from build123d import *

# Parameters (mm, degrees)
SKETCH1_W           = 9.849999945
SKETCH1_H           = 0.849999995
BOSS_EXTRUDE1_DEPTH = 10
BOSS_EXTRUDE2_DEPTH = 0.849999995
BOSS_EXTRUDE3_DEPTH = 0.150000005


with BuildPart() as part:
    # Sketch1 → Boss-Extrude1 (new body)
    with BuildSketch(Plane.XY):
        with Locations((2.94e-07, -2.739426966)):
            Rectangle(SKETCH1_W, SKETCH1_H)
    extrude(amount=BOSS_EXTRUDE1_DEPTH)

    # Sketch3 → Boss-Extrude2 (add)
    with BuildSketch(Plane.XZ.offset(3.164426964)):
        Polygon((-4.924999678, 0), (-4.924999678, 10), (-6.074999733, 10), (-6.074999733, 5.2), (-5.374999733, 4.6), (-5.374999733, 3.2), (-6.074999733, 3.2), (-6.074999733, 0), align=None)
    extrude(amount=-BOSS_EXTRUDE2_DEPTH)

    # Sketch4 → Boss-Extrude3 (add)
    with BuildSketch(Plane.XZ.offset(3.164426964)):
        with BuildLine():
            Line((-6.074999733, 10), (4.925000267, 10))
            Line((4.925000267, 10), (4.925000267, 8.5))
            ThreePointArc((4.925000267, 8.5), (-0.574999733, 8.25), (-6.074999733, 8.5))
            Line((-6.074999733, 8.5), (-6.074999733, 10))
        make_face()
    extrude(amount=BOSS_EXTRUDE3_DEPTH)


solid = part.part
Could you check a few things on this model? Use its own coordinates, in mm. Round coordinates to 2 decimals unless told otherwise and drop trailing zeros. Write each loop counter-clockwise with the first axis right and the second up, starting at its lowest first coordinate (ties: lowest second). Pieces come first, ordered by that corner, then holes. Notation, with made-up numbers: (24, 74) -> (71, 74) arc R23 ccw to (71, 103) -> close; hole circle Ø5 at (52, 11.25). An arc over 180 degrees is marked (long way). Use a Markdown table: item, result.
1. If we section it at D-D (x = -4.25): List the corners of the cut face in (y, z) for me, then the cut area to 3 significant figures.
Answer key:
| item | result |
|---|---|
| outline | (-3.31, 8.36) -> (-3.16, 8.36) -> (-3.16, 0) -> (-2.31, 0) -> (-2.31, 10) -> (-3.31, 10) -> close |
| area | 8.75 mm^2 |
2. If we section it at C-C (z = 6.5): List the corners of the cut face in (x, y) for me (3 decimals).
Answer key:
| item | result |
|---|---|
| outline | (-6.075, -3.164) -> (4.925, -3.164) -> (4.925, -2.314) -> (-6.075, -2.314) -> close |
3. If we section it at A-A (x = 1): List the corners of the cut face in (y, z) for me, then the cut area to 3 significant figures.
Answer key:
| item | result |
|---|---|
| outline | (-3.31, 8.27) -> (-3.16, 8.27) -> (-3.16, 0) -> (-2.31, 0) -> (-2.31, 10) -> (-3.31, 10) -> close |
| area | 8.76 mm^2 |
4. Please list where these lines run through material, in increasing order: probe 1 along Y at (x, z) = (-2.5, 4); probe 2 along Z at (x, y) = (-5.5, -2.7); probe 3 along X at (y, z) = (-3.1, 3.5) (3 decimals).
Answer key:
| item | result |
|---|---|
| probe 1 | y = -3.16 to -2.31 |
| probe 2 | z = 0 to 3.2, 4.71 to 10 |
| probe 3 | x = -5.375 to 4.925 |
5. If we section it at B-B (z = 5): List the corners of the cut face in (x, y) for me (3 decimals), then the cut area to 3 significant figures.
Answer key:
| item | result |
|---|---|
| outline | (-5.842, -3.164) -> (4.925, -3.164) -> (4.925, -2.314) -> (-5.842, -2.314) -> close |
| area | 9.15 mm^2 |
6. We'd pull the mould along Z, two halves only. Please class faces 1 (the face through (-1, -3, 10)), 2 (the face through (-1, -3, 0)), 3 (the face through (-5.375, -3, 4)): +Z half, -Z half, draft (parallel to the pull), parting line (faces both ways), or undercut.
Answer key:
| item | result |
|---|---|
| face 1 | +Z half |
| face 2 | -Z half |
| face 3 | undercut |
